Here's how the part is built. I have some questions about the finished solid (model axes, mm). A direction names the side the tool comes from. Coordinates: 2 decimals unless noted, no trailing zeros. Write each loop counter-clockwise with the first axis right and the second up, starting at its lowest first coordinate (ties: lowest second). Pieces come first, ordered by that corner, then holes. Notation, with made-up numbers: (75.25, 28.25) -> (120.25, 28.25) arc R16 ccw to (120.25, 49.25) -> close; hole circle Ø4 at (58, -16.5). An arc over 180 degrees is marked (long way). Put each result on its own line as item: value. Start each with the question number.
Item 1: If we mould it in two halves opening along X, with no side actions, what happens to faces 1 (the face through (-38.563, -7, 43)), 2 (the face through (348, -15, 42)), 3 (the face through (707.437, -7, 42))? For each: released by +X, released by -X, zero draft, split by the parting line, or undercut.
Item 2: I want a section at B-B, the plane y = -5.25. List the corners of the cut face in (x, z) for me, then the cut area to 3 significant figures.
Item 3: I want a section at A-A, the plane z = 47. List the corners of the cut face in (x, y) for me, then the cut area to 3 significant figures.
Item 4: I need wall thicknesses on line 1 (X direction, y = -9.75, z = 19.5); line 2 (X direction, y = -4.25, z = 68); line 3 (X direction, y = -10.25, z = 73). Which ranges of each line are inside material? Lowest first, please. Write a range as [from, to].
Item 5: On a 3-axis mill with a long thin cutter (end or side, diameter ignored), from which of +Z, -Z, +X, -X, +Y, -Y can I reach the whole of each face in a straight line? I mean faces 4 (the face through (348, 0, 42)), 5 (the face through (-4.563, -7, 42)). Say none if no direction works.
from build123d import *

# Parameters (mm, degrees)
CROQUIS1_W              = 785
CROQUIS1_H              = 100
SALIENTE_EXTRUIR1_DEPTH = 15
CROQUIS5_R              = 4.25
CORTAR_EXTRUIR4_DEPTH   = 16
CORTAR_EXTRUIR5_DEPTH   = 16


with BuildPart() as part:
    # Croquis1 → Saliente-Extruir1 (new body)
    with BuildSketch(Plane(origin=(0, 0, 0), x_dir=(1, 0, 0), z_dir=(0, 1, 0))):
        with Locations((353.936588921, -42.333090379)):
            Rectangle(CROQUIS1_W, CROQUIS1_H)
    extrude(amount=-SALIENTE_EXTRUIR1_DEPTH)

    # Croquis5 → Cortar-Extruir4 (cut, through all)
    with BuildSketch(Plane(origin=(0, 0, 0), x_dir=(1, 0, 0), z_dir=(0, 1, 0))):
        with Locations((258.936588921, -67.333090379)):
            Circle(CROQUIS5_R)
        with Locations((448.92606348, -69.332979585)):
            Circle(CROQUIS5_R)
    extrude(amount=-CORTAR_EXTRUIR4_DEPTH, mode=Mode.SUBTRACT)

    # Croquis6 → Cortar-Extruir5 (cut, through all)
    with BuildSketch(Plane(origin=(0, 0, 0), x_dir=(1, 0, 0), z_dir=(0, 1, 0))):
        with BuildLine():
            Line((717.436588921, -72.333090379), (717.436588921, -12.333090379))
            ThreePointArc((717.436588921, -12.333090379), (712.436588921, -7.333090379), (707.436588921, -12.333090379))
            Line((707.436588921, -12.333090379), (707.436588921, -72.333090379))
            ThreePointArc((707.436588921, -72.333090379), (712.436588921, -77.333090379), (717.436588921, -72.333090379))
        make_face()
        with BuildLine():
            Line((-4.563411079, -12.333090379), (-4.563411079, -72.333090379))
            ThreePointArc((-4.563411079, -72.333090379), (-9.563411079, -77.333090379), (-14.563411079, -72.333090379))
            Line((-14.563411079, -72.333090379), (-14.563411079, -12.333090379))
            ThreePointArc((-14.563411079, -12.333090379), (-9.563411079, -7.333090379), (-4.563411079, -12.333090379))
        make_face()
    extrude(amount=-CORTAR_EXTRUIR5_DEPTH, mode=Mode.SUBTRACT)


solid = part.part
Calculated:
1. face 1: released by -X
1. face 2: zero draft
1. face 3: undercut
2. outline: (-38.56, -7.67) -> (746.44, -7.67) -> (746.44, 92.33) -> (-38.56, 92.33) -> close; hole (-14.56, 12.33) arc R5 ccw to (-4.56, 12.33) -> (-4.56, 72.33) arc R5 ccw to (-14.56, 72.33) -> close; hole circle Ø8.5 at (258.94, 67.33); hole circle Ø8.5 at (448.93, 69.33); hole (707.44, 12.33) arc R5 ccw to (717.44, 12.33) -> (717.44, 72.33) arc R5 ccw to (707.44, 72.33) -> close
2. area: 77,000 mm2
3. outline: (-38.56, -15) -> (-14.56, -15) -> (-14.56, 0) -> (-38.56, 0) -> close; (-4.56, -15) -> (707.44, -15) -> (707.44, 0) -> (-4.56, 0) -> close; (717.44, -15) -> (746.44, -15) -> (746.44, 0) -> (717.44, 0) -> close
3. area: 11,500 mm2
4. line 1: x = [-38.56, -14.56], [-4.56, 707.44], [717.44, 746.44]
4. line 2: x = [-38.56, -14.56], [-4.56, 254.74], [263.13, 444.89], [452.96, 707.44], [717.44, 746.44]
4. line 3: x = [-38.56, -14.52], [-4.61, 446.78], [451.07, 707.48], [717.39, 746.44]
5. face 4: +Z, -Z, +X, -X, +Y
5. face 5: +Y, -Y
